```python
from build123d import *

# Parameters (mm, degrees)
F1_DEPTH = 22
F2_R     = 2.49999
F3_SIZE  = 2.5
F4_R     = 2.49999


# Not quite as in the source:
# - a fillet or chamfer is up to 0.001 mm smaller than in the source, because OpenCascade refuses the exact size


with BuildPart() as f1:
    # F0 (on Top) → F1 (new body)
    with BuildSketch(Plane.XY):
        Polygon((0, -40), (0, 0), (22.8, 0), (22.8, -40), (27.8, -40), (27.8, 0), (72.8, 0), (72.8, 13.6540349229), (67.8, 13.6540349229), (67.8, 5), (-5, 5), (-5, -40), align=None)
    extrude(amount=F1_DEPTH)

    # F2 (radius 2.5 in the source; OpenCascade refuses exactly that, so slightly less here)
    f2_edges = [f1.edges().sort_by_distance(p)[0] for p in [
        (72.8, 0, 11),
        (27.8, 0, 11),
        (67.8, 5, 11),
        (67.8, 13.654035, 11),
        (72.8, 13.654035, 11),
        (-5, 5, 11),
        (-5, -40, 11),
        (0, -40, 11),
    ]]
    fillet(f2_edges, radius=F2_R)

    # F3
    f3_edges = [f1.edges().sort_by_distance(p)[0] for p in [
        (27.8, -40, 11),
    ]]
    chamfer(f3_edges, length=F3_SIZE)

    # F4 (radius 2.5 in the source; OpenCascade refuses exactly that, so slightly less here)
    f4_edges = [f1.edges().sort_by_distance(p)[0] for p in [
        (22.8, -40, 11),
    ]]
    fillet(f4_edges, radius=F4_R)


solid = f1.part
```
Geometry: final body of the model. Coordinates: model frame, mm. A direction names the side the tool comes from. Round coordinates to 2 decimals unless told otherwise and drop trailing zeros. Write each loop counter-clockwise with the first axis right and the second up, starting at its lowest first coordinate (ties: lowest second). Pieces come first, ordered by that corner, then holes. Notation, with made-up numbers: M 59,77 L 113,77 A11 cw 113,88 Z; hole C -20,66 d2. An arc over 180 degrees is marked long. Answer in a Markdown table with one row per item. Add a question column.
(1) Cut plane A-A, the plane y = -17.5. Return the cut outline in (x, z).
(2) Ray query, L1, parallel to X at y = -19.5, z = 1.25; L2, parallel to Y at x = 57.5, z = 2; L3, parallel to X at y = 10, z = 19.75. Return the intervals inside material, ascending.
(3) Draft query along X for faces 6 (the face through (27.8, -20, 11)), 7 (the face through (25, -7, 22)), 8 (the face through (22.8, -18, 11)), 9 (the face through (-4.287, -39.248, 11.154)). Return one class per face: pulls with the +X half, pulls with the -X half, needs draft (parallel to the pull), parting line crosses it, or undercut.
(4) Contact query for flat-ended pins moving along their axis: pin 1 (6 mm diameter, centred on x = 17, z = 8.5, fed in from +Y); pin 2 (1.5 mm diameter, centred on x = 50.5, z = 14, fed in from -Y); pin 3 (10 mm diameter, centred on x = 37, y = -12.5, fed in from -Z); pin 4 (3 mm diameter, centred on y = 9, z = 10.5, fed in from -X). Output: stop coordinate, or through.
(5) Cut plane C-C, the plane x = 14. Return the cut outline in (y, z).
(6) Reachability of faces 1 (the face through (50, 0, 11)), 2 (the face through (11, 0, 11)), 3 (the face through (72.09, 12.9, 11.15)), 4 (the face through (25, -7, 0)), 5 (the face through (67.8, 9, 11)) from +Z, -Z, +X, -X, +Y, -Y: full face, straight path, thin tool, end or side. Return the list, or none.
(7) Cut plane D-D, the plane x = 26.5. Return the cut outline in (y, z), then the cut area to 3 significant figures.
Established:
| question | item | result |
|---|---|---|
| 1 | outline | M -5,0 L 0,0 L 0,22 L -5,22 Z; M 22.8,0 L 27.8,0 L 27.8,22 L 22.8,22 Z |
| 2 | L1 | -5 to 0, 22.8 to 27.8 |
| 2 | L2 | 0 to 5 |
| 2 | L3 | 67.8 to 72.8 |
| 3 | face 6 | pulls with the +X half |
| 3 | face 7 | needs draft |
| 3 | face 8 | undercut |
| 3 | face 9 | pulls with the -X half |
| 4 | pin 1 | y = 5 |
| 4 | pin 2 | y = 0 |
| 4 | pin 3 | through |
| 4 | pin 4 | x = 67.8 |
| 5 | outline | M 0,0 L 5,0 L 5,22 L 0,22 Z |
| 6 | face 1 | +Z, -Z, +X, -Y |
| 6 | face 2 | +Z, -Z, -Y |
| 6 | face 3 | +Z, -Z, +X, +Y |
| 6 | face 4 | -Z, +X, -X, +Y, -Y |
| 6 | face 5 | +Z, -Z, -X, +Y |
| 7 | outline | M -38.8,0 L 5,0 L 5,22 L -38.8,22 Z |
| 7 | area | 964 mm² |
